Part print with two shaded views. Sizes in mm from the minimum x, y, z corner. Give positions to 0.01 mm unless a question says otherwise; leave off trailing zeros. Order: outer loops, then holes, each group sorted by start corner. A loop starts at its lowest first (then second) coordinate and runs counter-clockwise, first axis right, second up. Notation, with made-up numbers: (-16, -22) -> (24, -22) arc R19 cw to (24, 8) -> close; hole circle Ø5 at (61, 10.25). An arc over 180 degrees is marked (long way). Write item = value, one per line. Start each with the question number.
Item 1: Band-saw the part on C-C on x = 38.5. Write the cut outline in (y, z), plus the area to 3 significant figures.
Item 2: Band-saw the part on A-A on y = 10. Write the cut outline in (x, z).
Item 3: Drill centre lines: line 1 along X through (y, z) = (10.75, 2.55); line 2 along Y through (x, z) = (6, 1.4); line 3 along Y through (x, z) = (38.5, 0.5). Where is each one in solid material? Low to high.
Item 4: Band-saw the part on B-B on z = 2.6. Write the cut outline in (x, y).
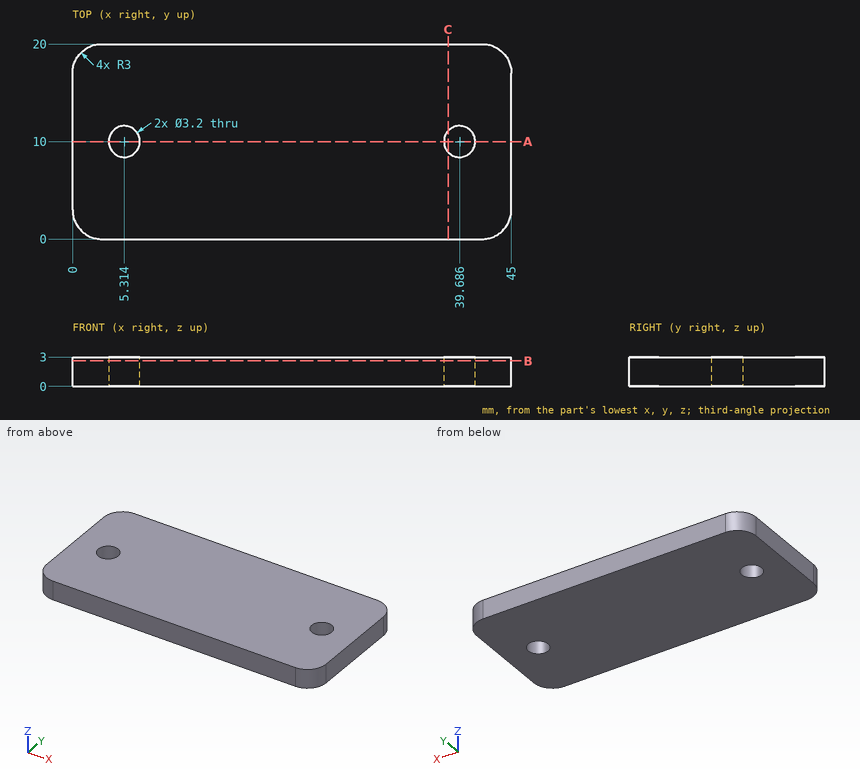
Values found:
q1.outline = (0, 0) -> (8.93, 0) -> (8.93, 3) -> (0, 3) -> close; (11.07, 0) -> (20, 0) -> (20, 3) -> (11.07, 3) -> close
q1.area = 53.6 mm^2
q2.outline = (0, 0) -> (3.71, 0) -> (3.71, 3) -> (0, 3) -> close; (6.91, 0) -> (38.09, 0) -> (38.09, 3) -> (6.91, 3) -> close; (41.29, 0) -> (45, 0) -> (45, 3) -> (41.29, 3) -> close
q3.line_1 = 0 to 3.9, 6.73 to 38.27, 41.1 to 45
q3.line_2 = 0 to 8.55, 11.45 to 20
q3.line_3 = 0 to 8.93, 11.07 to 20
q4.outline = (0, 3) arc R3 ccw to (3, 0) -> (42, 0) arc R3 ccw to (45, 3) -> (45, 17) arc R3 ccw to (42, 20) -> (3, 20) arc R3 ccw to (0, 17) -> close; hole circle Ø3.2 at (5.31, 10); hole circle Ø3.2 at (39.69, 10)
